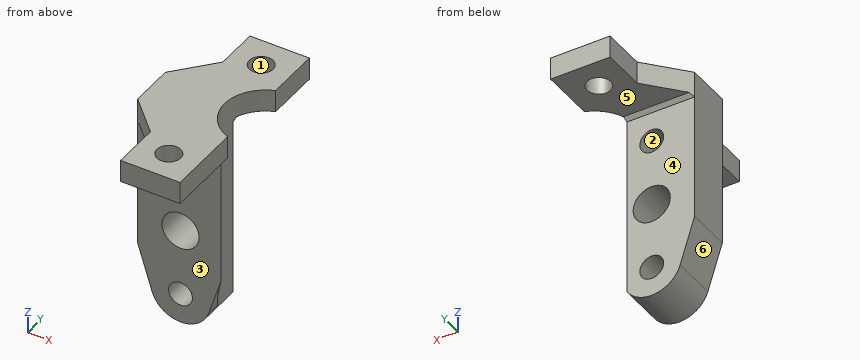
```python
from build123d import *

# Parameters (mm, degrees)
SKETCH_1_W               = 8
SKETCH_1_H               = 28
EXTRUDE_1_DEPTH          = 3
EXTRUDE_2_DEPTH          = 3
EXTRUDE_2_DEPTH_BACK     = 3
SKETCH_2_R               = 1.6
SKETCH_2_R_2             = 2.5
CUT_EXTRUDE_1_DEPTH      = 43.561738686
CUT_EXTRUDE_1_DEPTH_BACK = 43.561738686
SKETCH_3_R               = 5.5
EXTRUDE_3_DEPTH          = 3
SKETCH_6_R               = 1.6
CUT_EXTRUDE_2_DEPTH      = 41.5401234
CHAMFER_1_SIZE           = 0.5


with BuildPart() as part:
    # Эскиз1 → Бобышка-Вытянуть1 (new body)
    with BuildSketch(Plane.XY):
        with Locations((-4, -14)):
            Rectangle(SKETCH_1_W, SKETCH_1_H)
    extrude(amount=EXTRUDE_1_DEPTH)

    # Эскиз2 → Бобышка-Вытянуть2 (add, two sides: drawn at the far end of the back side and taken through both)
    with BuildSketch(Plane(origin=(0, -14, 0), x_dir=(1, 0, 0), z_dir=(0, 1, 0)).offset(-EXTRUDE_2_DEPTH_BACK)):
        with BuildLine():
            Line((-1, 9.5), (-1, 17.5))
            Line((-1, 17.5), (-2.955024535, 23.702481686))
            ThreePointArc((-2.955024535, 23.702481686), (-6.77, 26.5), (-10.584975465, 23.702481686))
            Line((-10.584975465, 23.702481686), (-12.54, 17.5))
            Line((-12.54, 17.5), (-12.54, 9.5))
            Line((-12.54, 9.5), (-12.54, -3))
            Line((-12.54, -3), (0, -3))
            Line((0, -3), (0, 0))
            Line((0, 0), (-1, 0))
            Line((-1, 0), (-1, 9.5))
        make_face()
        with Locations(Location((-6.77, 22.5, 0), (0, 0, 180))):
            Circle(SKETCH_2_R, mode=Mode.SUBTRACT)
        with Locations(Location((-6.77, 4.5, 0), (0, 0, 180))):
            Circle(SKETCH_2_R, mode=Mode.SUBTRACT)
        with Locations(Location((-6.77, 13.5, 0), (0, 0, 180))):
            Circle(SKETCH_2_R_2, mode=Mode.SUBTRACT)
    extrude(amount=EXTRUDE_2_DEPTH + EXTRUDE_2_DEPTH_BACK)

    # Эскиз3 → Вырез-Вытянуть1 (cut, two sides: drawn at the far end of the back side and taken through both)
    with BuildSketch(Plane.XY.offset(3).offset(-CUT_EXTRUDE_1_DEPTH_BACK)):
        with Locations((1.85, -12.5)):
            Circle(SKETCH_3_R)
    extrude(amount=CUT_EXTRUDE_1_DEPTH + CUT_EXTRUDE_1_DEPTH_BACK, mode=Mode.SUBTRACT)

    # Эскиз4 → Бобышка-Вытянуть3 (add)
    with BuildSketch(Plane.XY.offset(3)):
        Polygon((-12.54, -11), (-8, -5.855638374), (-8, -21.54), (-12.54, -17), align=None)
    extrude(amount=-EXTRUDE_3_DEPTH)

    # Эскиз6 → Вырез-Вытянуть2 (cut, through all)
    with BuildSketch(Plane(origin=(0, 0, 0), x_dir=(-1, 0, 0), z_dir=(0, 0, -1))):
        with Locations((4, -4)):
            Circle(SKETCH_6_R)
        with Locations((4, -24)):
            Circle(SKETCH_6_R)
    extrude(amount=-CUT_EXTRUDE_2_DEPTH, mode=Mode.SUBTRACT)

    # Фаска1
    chamfer_1_edges = [part.edges().sort_by_distance(p)[0] for p in [
        (-6.92613883, -17, 0),
        (-7.990751311, -11, 0),
    ]]
    chamfer(chamfer_1_edges, length=CHAMFER_1_SIZE)


solid = part.part
```
The listing builds one solid part. Answer for the finished solid, in the listing's coordinates (mm). Face numbers are marked on the shaded views. A direction names the side the tool comes from. Give positions to 0.01 mm unless a question says otherwise; leave off trailing zeros. Loops run counter-clockwise (first coordinate to the right, second up) from the corner with the lowest first, then second, coordinate; pieces in that order, holes last. Notation, with made-up numbers: M 60,46 L 94,46 A23 cw 94,81 Z; hole C -26.75,-33.75 d1. An arc over 180 degrees is marked long. One line per item, written item: value.
Q1. Find the intervals of material crossed by line 1 (Y direction, x = -4, z = 1.65); line 2 (Z direction, x = -6.77, y = -14.2); line 3 (Y direction, x = -10.75, z = -14.25), in increasing order. Write a range as from..to.
Working result:
line 1: y = -28..-25.6, -22.4..-5.6, -2.4..0
line 2: z = -26.5..-24.1, -20.9..-16, -11..-6.1, -2.9..3
line 3: y = -17..-11
Q2. A cutting plane is placed at B-B on x = -6.77. Determine the outline of the cut face in (y, z).
Working result:
outline: M -28,0 L -17.5,0 L -17,-0.5 L -17,-2.9 L -11,-2.9 L -11,-0.5 L -10.5,0 L 0,0 L 0,3 L -28,3 Z; M -17,-26.5 L -11,-26.5 L -11,-24.1 L -17,-24.1 Z; M -17,-20.9 L -11,-20.9 L -11,-16 L -17,-16 Z; M -17,-11 L -11,-11 L -11,-6.1 L -17,-6.1 Z
Q3. Flat-ended cylindrical pins translate along their axes: P1, Ø5, axis at x = -6.77, z = -22.5, coming from the +Y side; P2, Ø2.5, axis at x = -4, y = -24, coming from the -Z side; P3, Ø5, axis at x = -5, y = -23.5, coming from the -Z side; P4, Ø2.5, axis at y = -3, z = 1, coming from the -X side. Find the tip coordinate at first contact, or state that the pin passes through.
Working result:
P1: stops at y = -11
P2: passes through
P3: stops at z = 0
P4: stops at x = -8
Q4. A cutting plane is placed at C-C on z = -4.5. Determine the outline of the cut face in (x, y).
Working result:
outline: M -12.54,-17 L -8.37,-17 L -8.37,-11 L -12.54,-11 Z; M -5.17,-17 L -1.31,-17 A5.5 cw -3.44,-11 L -5.17,-11 Z
Q5. A cutting plane is placed at D-D on y = -14.75. Determine the outline of the cut face in (x, z).
Working result:
outline: M -12.54,-17.5 L -10.58,-23.7 A4 ccw -3.17,-24.24 L -3.17,3 L -12.54,3 Z; hole C -6.77,-13.5 d5; hole C -6.77,-22.5 d3.2; hole C -6.77,-4.5 d3.2
Q6. A cutting plane is placed at A-A on y = -24. Determine the outline of the cut face in (x, z).
Working result:
outline: M -8,0 L -5.6,0 L -5.6,3 L -8,3 Z; M -2.4,0 L 0,0 L 0,3 L -2.4,3 Z
Q7. For the marked faces 5 and 6, determine the directions among +Z, -Z, +X, -X, +Y, -Y from which every point of the face is accessible in a straight line to the end or side of a thin tool.
Working result:
face 5: -Z, +X, -X, +Y
face 6: -Z, -X, +Y, -Y
Q8. Determine the mould class of the marked faces 1, 2, 3 and 4 for opening direction Y: +Y half, -Y half, draft (parallel to the pull), parting line (faces both ways), or undercut.
Working result:
face 1: undercut
face 2: draft
face 3: -Y half
face 4: +Y half
